Verification items for this drawing (mm, ordinates from the low corner). A direction names the side the tool comes from. Round coordinates to 2 decimals unless told otherwise and drop trailing zeros. Order: outer loops, then holes, each group sorted by start corner. A loop starts at its lowest first (then second) coordinate and runs counter-clockwise, first axis right, second up. Notation, with made-up numbers: (30.25, 13) - (50.25, 13) arc R19 ccw to (50.25, 32) - close; hole circle Ø9 at (41, 60.25). An arc over 180 degrees is marked (long way). Return JSON: item names as keys, results as strings. Group by question number.
Q1. Tool access check on the marked faces 4, 5 and 6. Record the directions out of +Z, -Z, +X, -X, +Y, -Y that give a thin tool (end or side, any length) a straight path to the whole face; none if there is none.
Q2. Sectioned sample at C-C, the plane z = 2.75. Record the cut outline in (x, y), then the cut area to 3 significant figures.
Q3. Sectioned sample at B-B, the plane x = 9.25. Record the cut outline in (y, z), then the cut area to 3 significant figures.
Q4. Material ranges on line 1 along Z through (x, y) = (7.75, 14); line 2 along X through (y, z) = (14.5, 14.25) (1 decimal); line 3 along Z through (x, y) = (14.25, 13.5) (1 decimal), recorded low to high.
Q5. Draft check along X on the marked faces 1, 2 and 3. Enter one of: pulls with the +X half, pulls with the -X half, needs draft (parallel to the pull), parting line crosses it, or undercut.
Q6. Gauge pin test, flat ends, axial feed: pin 1 Ø7.5 at (x, y) = (8, 4.5) entering from +Z; pin 2 Ø6 at (x, z) = (4.5, 3.5) entering from -Y; pin 3 Ø5 at (y, z) = (32.5, 12.5) entering from +X; pin 4 Ø3 at (x, z) = (12.5, 9) entering from +Y. Record the tip position at first contact, or that the pin passes through.
Q7. Sectioned sample at A-A, the plane y = 22. Record the cut outline in (x, z).
Q8. Sectioned sample at D-D, the plane x = 13. Record the cut outline in (y, z) (1 decimal).
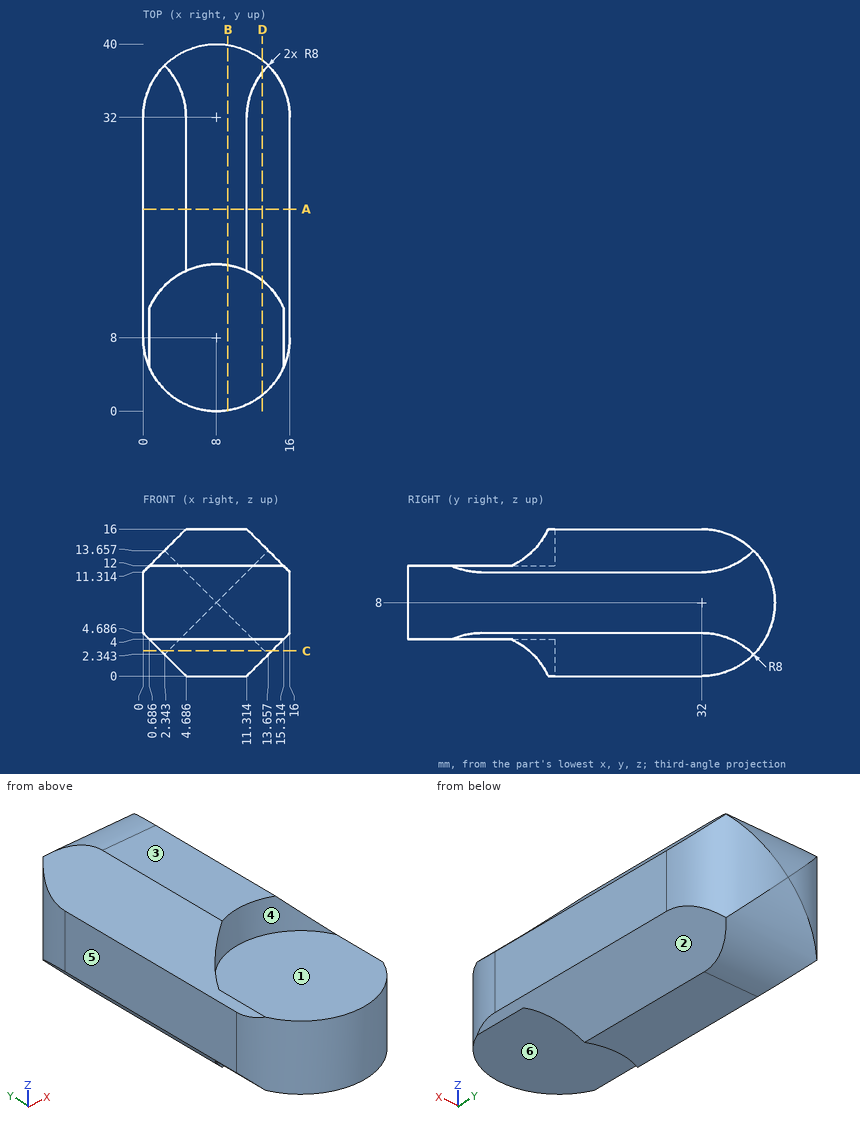
Reply:
{
 "1": {"face 4": "+Z, -Y", "face 5": "+Z, -Z, -X, +Y, -Y", "face 6": "-Z, -Y"},
 "2": {"outline": "(1.94, 13.22) arc R8 cw to (14.06, 13.22) - (14.06, 37.22) arc R8 ccw to (13.25, 38.04) - (2.75, 38.04) arc R8 ccw to (1.94, 37.22) - close", "area": "277 mm^2"},
 "3": {"outline": "(0.1, 4) - (15.9, 4) - (15.9, 0) - (32, 0) arc R8 ccw to (39.9, 6.75) - (39.9, 9.25) arc R8 ccw to (32, 16) - (15.9, 16) - (15.9, 12) - (0.1, 12) - close", "area": "484 mm^2"},
 "4": {"line 1": "4 to 12", "line 2": "2.9 to 3.3, 12.7 to 13.1", "line 3": "2.9 to 13.1"},
 "5": {"face 1": "undercut", "face 2": "pulls with the +X half", "face 3": "needs draft"},
 "6": {"pin 1": "z = 12", "pin 2": "y = 0.02", "pin 3": "x = 16", "pin 4": "y = 39.42"},
 "7": {"outline": "(0, 4.69) - (4.69, 0) - (11.31, 0) - (16, 4.69) - (16, 11.31) - (11.31, 16) - (4.69, 16) - (0, 11.31) - close"},
 "8": {"outline": "(1.8, 4) - (14.2, 4) - (14.2, 1.7) - (36.9, 1.7) arc R8 ccw to (38.2, 3) - (38.2, 13) arc R8 ccw to (36.9, 14.3) - (14.2, 14.3) - (14.2, 12) - (1.8, 12) - close"}
}
